The figure shows three views and two pictorial views of one solid part (mm, origin at its lowest corner). Answer the questions. Give positions to 0.01 mm unless a question says otherwise; leave off trailing zeros. Loops run counter-clockwise (first coordinate to the right, second up) from the corner with the lowest first, then second, coordinate; pieces in that order, holes last. Notation, with made-up numbers: (-29, 74.25) - (-18, 74.25) arc R28 cw to (-18, 92.25) - close; hole circle Ø11 at (-24, -1). An arc over 180 degrees is marked (long way). Use CSV: the item, a comma, the result in double quotes.
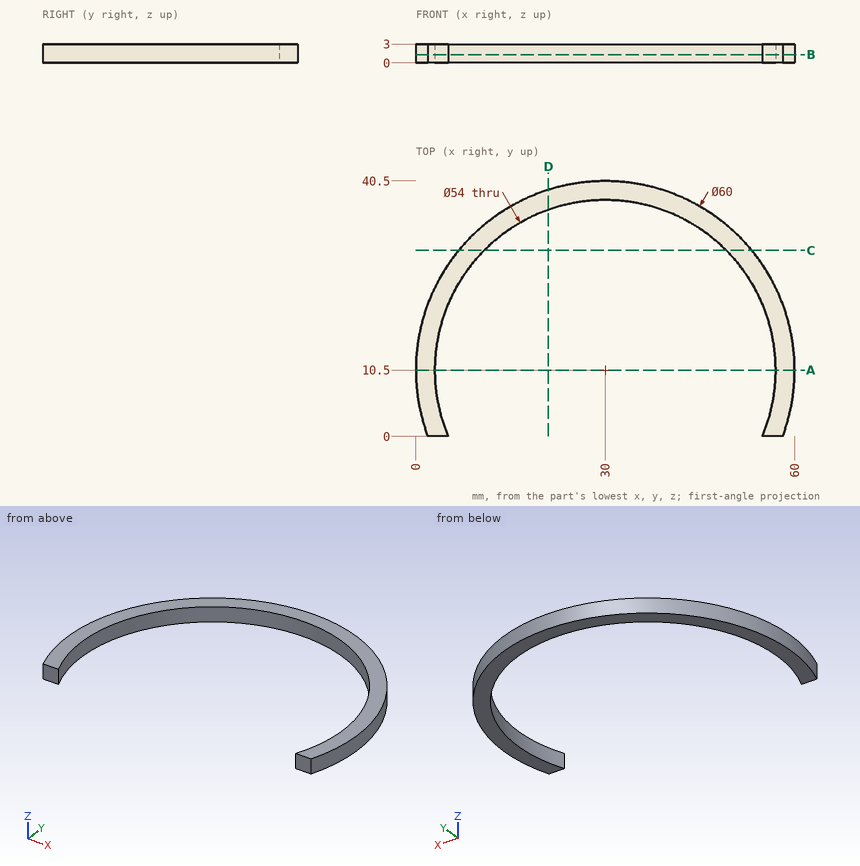
Item 1: A cutting plane is placed at C-C on y = 29.5. Determine the outline of the cut face in (x, z).
Determined:
outline,"(6.78, 0) - (10.82, 0) - (10.82, 3) - (6.78, 3) - close; (49.18, 0) - (53.22, 0) - (53.22, 3) - (49.18, 3) - close"
Item 2: A cutting plane is placed at D-D on x = 21. Determine the outline of the cut face in (y, z), and give its area (3 significant figures).
Determined:
outline,"(35.96, 0) - (39.12, 0) - (39.12, 3) - (35.96, 3) - close"
area,"9.49 mm²"
Item 3: A cutting plane is placed at B-B on z = 1.3. Determine the outline of the cut face in (x, y), and give its area (3 significant figures).
Determined:
outline,"(1.9, 0) - (5.13, 0) arc R27 cw (long way) to (54.87, 0) - (58.1, 0) arc R30 ccw (long way) to start"
area,"333 mm²"
Item 4: Find the intervals of material crossed by line 1 (X direction, y = 10.5, z = 1.15); line 2 (Y direction, x = 30, z = 0.95); line 3 (X direction, y = 34.5, z = 2.25), in increasing order.
Determined:
line 1,"x = 0 to 3, 57 to 60"
line 2,"y = 37.5 to 40.5"
line 3,"x = 12 to 17.63, 42.37 to 48"
Item 5: Given P1, Ø6, axis at x = 11.5, y = 20.5, coming from the +Z side, flat-ended and moving along its own axis, determine where the tip first touches the part or whether it passes through.
Determined:
P1,"passes through"
Item 6: A cutting plane is placed at A-A on y = 10.5. Determine the outline of the cut face in (x, z), and give its area (3 significant figures).
Determined:
outline,"(0, 0) - (3, 0) - (3, 3) - (0, 3) - close; (57, 0) - (60, 0) - (60, 3) - (57, 3) - close"
area,"18.0 mm²"
